from build123d import *

# Parameters (mm, degrees)
SKETCH1_W           = 10
SKETCH1_H           = 10
BOSS_EXTRUDE1_DEPTH = 3
SKETCH2_W           = 13
SKETCH2_H           = 10
BOSS_EXTRUDE2_DEPTH = 3
SKETCH3_R           = 1.6
CUT_EXTRUDE1_DEPTH  = 4
SKETCH4_R           = 1.6
CUT_EXTRUDE2_DEPTH  = 4


with BuildPart() as part:
    # Sketch1 → Boss-Extrude1 (new body)
    with BuildSketch(Plane.XY):
        with Locations((5, -5)):
            Rectangle(SKETCH1_W, SKETCH1_H)
    extrude(amount=BOSS_EXTRUDE1_DEPTH)

    # Sketch2 → Boss-Extrude2 (add)
    with BuildSketch(Plane(origin=(10, 0, 0), x_dir=(0, 0, -1), z_dir=(1, 0, 0))):
        with Locations((-6.5, -5)):
            Rectangle(SKETCH2_W, SKETCH2_H)
    extrude(amount=BOSS_EXTRUDE2_DEPTH)

    # Sketch3 → Cut-Extrude1 (cut, through all)
    with BuildSketch(Plane.XY.offset(3)):
        with Locations((5, -2.5)):
            Circle(SKETCH3_R)
        with Locations((5, -7.5)):
            Circle(SKETCH3_R)
    extrude(amount=-CUT_EXTRUDE1_DEPTH, mode=Mode.SUBTRACT)

    # Sketch4 → Cut-Extrude2 (cut, through all)
    with BuildSketch(Plane.ZY.offset(-10)):
        with Locations((8, -2.5)):
            Circle(SKETCH4_R)
        with Locations((8, -7.5)):
            Circle(SKETCH4_R)
    extrude(amount=-CUT_EXTRUDE2_DEPTH, mode=Mode.SUBTRACT)


solid = part.part
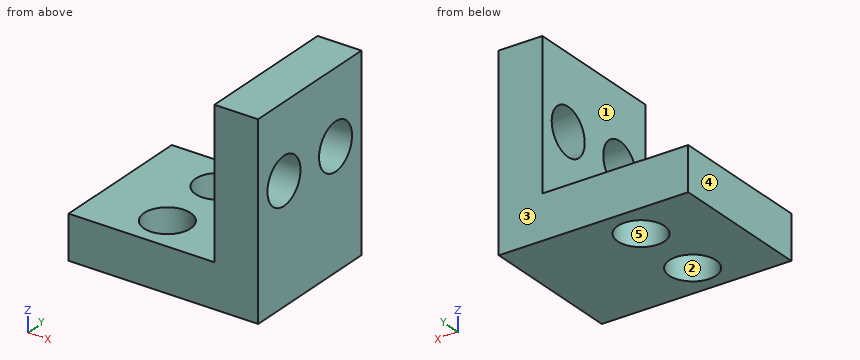
Work out the finished part from the listing and answer in its coordinate system (mm). Face numbers are marked on the shaded views. A direction names the side the tool comes from. Coordinates: 2 decimals unless noted, no trailing zeros. Order: outer loops, then holes, each group sorted by start corner. A loop starts at its lowest first (then second) coordinate and runs counter-clockwise, first axis right, second up. Notation, with made-up numbers: (-10, 17.5) - (13, 17.5) arc R25 cw to (13, 52.5) - close; hole circle Ø11 at (80, -12.5). An arc over 180 degrees is marked (long way). Put each result on its own line as item: value. Start each with the question number.
1) For a pull along X with two mould halves and no side action, classify the marked faces 3, 4 and 5 as released by +X, released by -X, zero draft, split by the parting line, or undercut.
2) For the marked faces 1 and 2, determine the directions among +Z, -Z, +X, -X, +Y, -Y from which every point of the face is accessible in a straight line to the end or side of a thin tool.
3) Find section C-C (y = -2.5). Give the vertices of the cut face in (x, z), plus the area to 3 significant figures.
4) Find section D-D (x = 12). Give the vertices of the cut face in (y, z), plus the area to 3 significant figures.
5) Flat-ended cylindrical pins translate along their axes: pin 1 (3 mm diameter, centred on x = 5, y = -7.5, fed in from +Z); pin 2 (3 mm diameter, centred on y = -4.5, z = 5.5, fed in from -X); pin 3 (3.5 mm diameter, centred on x = 5, y = -2.5, fed in from +Z). Find the tip coordinate at first contact, or state that the pin passes through.
6) Find section B-B (x = 5). Give the vertices of the cut face in (y, z), plus the area to 3 significant figures.
7) Find the intervals of material crossed by line 1 (Y direction, x = 5, z = 0.75); line 2 (Y direction, x = 5.5, z = 2.5); line 3 (X direction, y = -3, z = 10.25), in increasing order. Write a range as from..to.
8) Find section A-A (z = 8). Give the vertices of the cut face in (x, y).
Results list:
1. face 3: zero draft
1. face 4: released by -X
1. face 5: undercut
2. face 1: +Z, -X, +Y, -Y
2. face 2: +Z, -Z
3. outline: (0, 0) - (3.4, 0) - (3.4, 3) - (0, 3) - close; (6.6, 0) - (13, 0) - (13, 6.4) - (10, 6.4) - (10, 3) - (6.6, 3) - close; (10, 9.6) - (13, 9.6) - (13, 13) - (10, 13) - close
3. area: 49.8 mm^2
4. outline: (-10, 0) - (0, 0) - (0, 13) - (-10, 13) - close; hole circle Ø3.2 at (-7.5, 8); hole circle Ø3.2 at (-2.5, 8)
4. area: 114 mm^2
5. pin 1: passes through
5. pin 2: stops at x = 10
5. pin 3: stops at z = 3
6. outline: (-10, 0) - (-9.1, 0) - (-9.1, 3) - (-10, 3) - close; (-5.9, 0) - (-4.1, 0) - (-4.1, 3) - (-5.9, 3) - close; (-0.9, 0) - (0, 0) - (0, 3) - (-0.9, 3) - close
6. area: 10.8 mm^2
7. line 1: y = -10..-9.1, -5.9..-4.1, -0.9..0
7. line 2: y = -10..-9.02, -5.98..-4.02, -0.98..0
7. line 3: x = 10..13
8. outline: (10, -10) - (13, -10) - (13, -9.1) - (10, -9.1) - close; (10, -5.9) - (13, -5.9) - (13, -4.1) - (10, -4.1) - close; (10, -0.9) - (13, -0.9) - (13, 0) - (10, 0) - close
